from build123d import *

# Parameters (mm, degrees)
SKETCH_1_W          = 158.45
SKETCH_1_H          = 150
EXTRUDE_1_DEPTH     = 2
SKETCH_2_R          = 82.5
CUT_EXTRUDE_1_DEPTH = 10
SKETCH_4_W          = 10
SKETCH_4_H          = 6
CUT_EXTRUDE_2_DEPTH = 10
FILLET_1_R          = 1.1
SKETCH_5_R          = 1.6
CUT_EXTRUDE_3_DEPTH = 10
CUT_EXTRUDE_4_DEPTH = 10
EXTRUDE_2_DEPTH     = 2
FILLET_2_R          = 1.5
FILLET_3_R          = 10
FILLET_4_R          = 3
CUT_EXTRUDE_5_DEPTH = 10


with BuildPart() as part:
    # 草图1 → 凸台-拉伸1 (new body)
    with BuildSketch(Plane.XY):
        Rectangle(SKETCH_1_W, SKETCH_1_H)
    extrude(amount=EXTRUDE_1_DEPTH)

    # 草图2 → 切除-拉伸1 (cut)
    with BuildSketch(Plane(origin=(0, 0, 0), x_dir=(-1, 0, 0), z_dir=(0, 0, -1))):
        with Locations((2.825, -130)):
            Circle(SKETCH_2_R)
    extrude(amount=-CUT_EXTRUDE_1_DEPTH, mode=Mode.SUBTRACT)

    # 草图4 → 切除-拉伸2 (cut)
    with BuildSketch(Plane(origin=(0, 0, 0), x_dir=(-1, 0, 0), z_dir=(0, 0, -1))):
        with Locations((79.225, -9)):
            Rectangle(SKETCH_4_W, SKETCH_4_H)
    extrude(amount=-CUT_EXTRUDE_2_DEPTH, mode=Mode.SUBTRACT)

    # 圆角1
    fillet_1_edges = [part.edges().sort_by_distance(p)[0] for p in [
        (-74.225, -12, 1),
        (-74.225, -6, 1),
    ]]
    fillet(fillet_1_edges, radius=FILLET_1_R)

    # 草图5 → 切除-拉伸3 (cut)
    with BuildSketch(Plane.XY.offset(2)):
        with Locations((76.225, 20)):
            Circle(SKETCH_5_R)
        with Locations((76.225, 0)):
            Circle(SKETCH_5_R)
        with Locations((-76.225, 45)):
            Circle(SKETCH_5_R)
        with Locations((-76.225, 25)):
            Circle(SKETCH_5_R)
    extrude(amount=-CUT_EXTRUDE_3_DEPTH, mode=Mode.SUBTRACT)

    # 草图6 → 切除-拉伸4 (cut)
    with BuildSketch(Plane.XY.offset(2)):
        with BuildLine():
            Line((-55.225, 65), (-70.225, 65))
            Line((-70.225, 65), (-70.225, -66.647888749))
            ThreePointArc((-70.225, -66.647888749), (-63.069899561, -59.80881767), (-55.225, -53.773429829))
            Line((-55.225, -53.773429829), (-55.225, 65))
        make_face()
        with BuildLine():
            Line((-32.225, 65), (-47.225, 65))
            Line((-47.225, 65), (-47.225, -48.852664862))
            ThreePointArc((-47.225, -48.852664862), (-39.870317713, -45.242142337), (-32.225, -42.296579314))
            Line((-32.225, -42.296579314), (-32.225, 65))
        make_face()
        with BuildLine():
            Line((-9, 65), (-24.225, 65))
            Line((-24.225, 65), (-24.225, -40.009500501))
            ThreePointArc((-24.225, -40.009500501), (-16.660508355, -38.540562496), (-9, -37.706341632))
            Line((-9, -37.706341632), (-9, 65))
        make_face()
    cut_extrude_4 = extrude(amount=-CUT_EXTRUDE_4_DEPTH, mode=Mode.SUBTRACT)

    # 镜向1: 切除-拉伸4 across plane
    add(cut_extrude_4.mirror(Plane(origin=(0, 0, 0), x_dir=(0, 0, 1), z_dir=(1, 0, 0))), mode=Mode.SUBTRACT)

    # 草图7 → 凸台-拉伸2 (add)
    with BuildSketch(Plane.XY.offset(2)):
        Polygon((-72.801882642, 63.463876356), (-11.576882642, -39.242465276), (-6.423117358, -36.170217988), (-67.648117358, 66.536123644), align=None)
        Polygon((67.648117358, 66.536123644), (6.423117358, -36.170217988), (11.576882642, -39.242465276), (72.801882642, 63.463876356), align=None)
    extrude(amount=-EXTRUDE_2_DEPTH)

    # 圆角2
    fillet_2_edges = [part.edges().sort_by_distance(p)[0] for p in [
        (-32.225, -42.296579314, 1),
        (-47.225, -48.852664862, 1),
        (-47.225, 65, 1),
        (-32.225, 65, 1),
        (-24.225, -40.009500501, 1),
        (-24.225, 65, 1),
        (-9, 65, 1),
        (70.225, -66.647888749, 1),
        (55.225, -53.773429829, 1),
        (55.225, 65, 1),
        (47.225, -48.852664862, 1),
        (32.225, -42.296579314, 1),
        (32.225, 65, 1),
        (47.225, 65, 1),
        (24.225, -40.009500501, 1),
        (9, 65, 1),
        (24.225, 65, 1),
        (-55.225, 45.696059365, 1),
        (-55.225, 33.978252617, 1),
        (-12.32407353, -37.989035425, 1),
        (-24.225, -18.024958336, 1),
        (-47.225, 20.558069145, 1),
        (-9, -31.847438258, 1),
        (-32.225, 7.113031883, 1),
        (-47.225, 32.275875893, 1),
        (-70.225, 59.141096626, 1),
        (-66.732407884, 65, 1),
        (70.225, 59.141096626, 1),
        (66.732407884, 65, 1),
        (32.225, 7.113031883, 1),
        (47.225, 32.275875893, 1),
        (55.225, 45.696059365, 1),
        (9, -31.847438258, 1),
        (24.225, -18.024958336, 1),
        (47.225, 20.558069145, 1),
        (55.225, 33.978252617, 1),
        (12.32407353, -37.989035425, 1),
        (-55.225, -53.773429829, 1),
        (-70.225, -66.647888749, 1),
        (-55.225, 65, 1),
    ]]
    fillet(fillet_2_edges, radius=FILLET_2_R)

    # 圆角3
    fillet_3_edges = [part.edges().sort_by_distance(p)[0] for p in [
        (-32.225, -4.604774864, 1),
        (-24.225, -6.307151588, 1),
        (24.225, -6.307151588, 1),
        (32.225, -4.604774864, 1),
    ]]
    fillet(fillet_3_edges, radius=FILLET_3_R)

    # 圆角4
    fillet_4_edges = [part.edges().sort_by_distance(p)[0] for p in [
        (58.666869381, -75, 1),
        (-64.316869381, -75, 1),
        (79.225, -75, 1),
        (-79.225, -75, 1),
        (-79.225, 75, 1),
        (79.225, 75, 1),
    ]]
    fillet(fillet_4_edges, radius=FILLET_4_R)

    # 草图10 → 切除-拉伸5 (cut)
    with BuildSketch(Plane.XY.offset(2)):
        with BuildLine():
            Line((3, 62), (3, -32.5))
            ThreePointArc((3, -32.5), (0, -35.5), (-3, -32.5))
            Line((-3, -32.5), (-3, 62))
            ThreePointArc((-3, 62), (0, 65), (3, 62))
        make_face()
    extrude(amount=-CUT_EXTRUDE_5_DEPTH, mode=Mode.SUBTRACT)


solid = part.part
Work out the finished part from the listing and answer in its coordinate system (mm). A direction names the side the tool comes from. Give positions to 0.01 mm unless a question says otherwise; leave off trailing zeros. Loops run counter-clockwise (first coordinate to the right, second up) from the corner with the lowest first, then second, coordinate; pieces in that order, holes last. Notation, with made-up numbers: (-19.75, 15.25) -> (18.25, 15.25) arc R16 cw to (18.25, 41.25) -> close; hole circle Ø6 at (75, 46). An arc over 180 degrees is marked (long way). Use a Markdown table: item, result. Add a question column.
1) Which of the six approach directions +Z, -Z, +X, -X, +Y, -Y give full straight-line access (tool end or side, diameter ignored) to faces 1 (the cylindrical face through (62.056, -58.951, 1.014)), 2 (the cylindrical face through (-3.778, -47.506, 0.986))?
2) Consider line 1 along X through (y, z) = (-40, 1.55) (3 decimals); line 2 along Y through (x, z) = (14, 1.35); line 3 along Y through (x, z) = (64.5, 0.8). Determine where each line is inside the solid, lowest interval first.
3) Each of these flat-tipped pins is pushed along its axis until it touches: P1, Ø3.5, axis at x = -76.225, y = 45, coming from the -Z side; P2, Ø1, axis at x = -60, z = 1.5, coming from the -Y side; P3, Ø3, axis at x = 57.5, y = -49.5, coming from the +Z side; P4, Ø0.6, axis at x = 42.5, z = 1, coming from the -Y side. Where does it stop, or does it pass through?
4) The part is cut by section B-B, the plane z = 0.75. Count the separate pieces of the cut face and the enclosed holes in it, plus the area to 3 significant figures.
5) For a pull along X with two mould halves and no side action, classify faces 3 (the flat face through (17.42, -29.44, 1.01)), 4 (the flat face through (-19, -16, 2)) as +X half, -X half, draft (parallel to the pull), parting line (faces both ways), or undercut.
6) The part is cut by section A-A, the plane x = 0. Determine the outline of the cut face in (y, z), plus the area to 3 significant figures.
Reported:
| question | item | result |
|---|---|---|
| 1 | face 1 | +Z, -Z |
| 1 | face 2 | +Z, -Z, -Y |
| 2 | line 1 | x = -79.225 to -70.225, -55.225 to -47.225, -32.225 to 32.225, 47.225 to 55.225, 70.225 to 79.225 |
| 2 | line 2 | y = -49.23 to -38.03, -35.18 to -23.46, 65 to 75 |
| 2 | line 3 | y = -75 to -61.06, 49.54 to 61.26, 64.94 to 75 |
| 3 | P1 | stops at z = 0 |
| 3 | P2 | stops at y = -71.01 |
| 3 | P3 | passes through |
| 3 | P4 | stops at y = -61.26 |
| 4 | separate pieces | 1 |
| 4 | enclosed holes | 17 |
| 4 | area | 11,700 mm^2 |
| 5 | face 3 | undercut |
| 5 | face 4 | draft |
| 6 | outline | (-47.55, 0) -> (-35.5, 0) -> (-35.5, 2) -> (-47.55, 2) -> close; (65, 0) -> (75, 0) -> (75, 2) -> (65, 2) -> close |
| 6 | area | 44.1 mm^2 |
